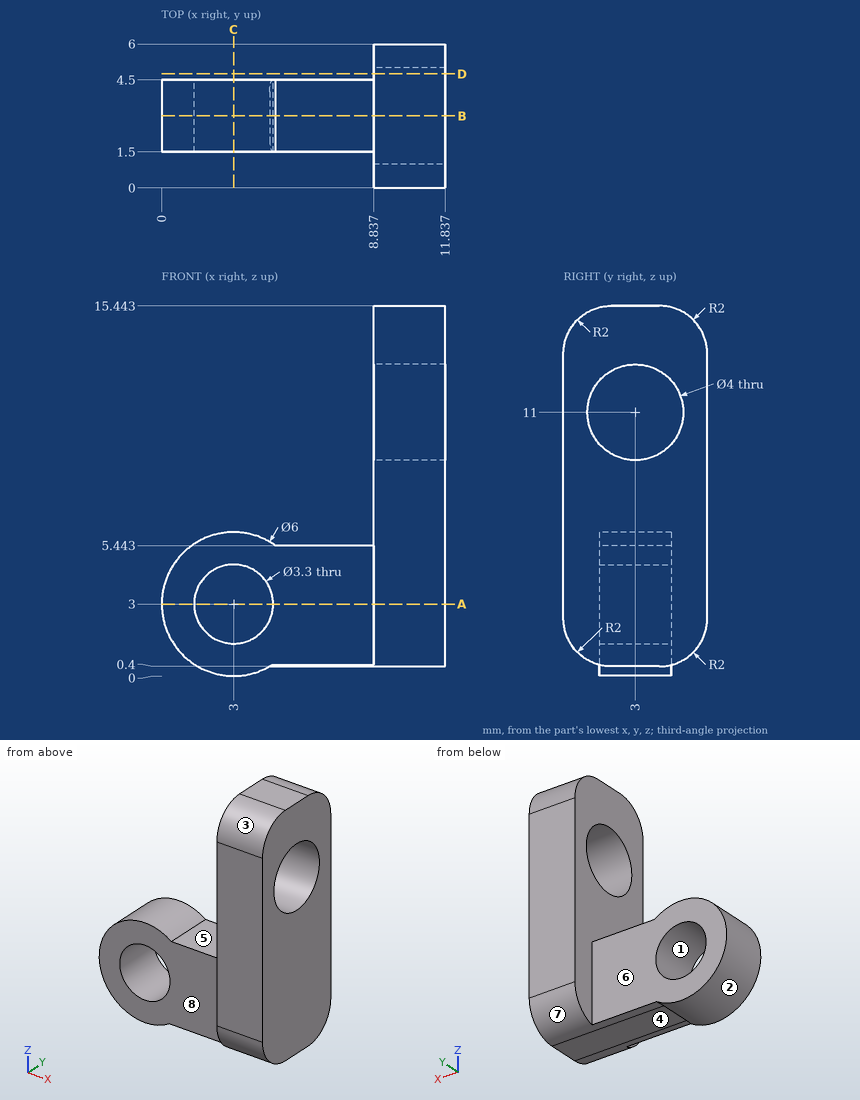
Geometry: see drawing. Coordinates: mm, zero at the bounding-box minimum. A direction names the side the tool comes from. Round coordinates to 2 decimals unless told otherwise and drop trailing zeros. Write each loop counter-clockwise with the first axis right and the second up, starting at its lowest first coordinate (ties: lowest second). Pieces come first, ordered by that corner, then holes. Notation, with made-up numbers: M 39,14 L 63,14 A38 ccw 63,52 Z; hole C 53.5,15 d1. An arc over 180 degrees is marked long. Answer in a Markdown table with one row per item. Add a question column.
(1) Ray query, L1, parallel to Z at x = 3, y = 3; L2, parallel to X at y = 4.25, z = 13; L3, parallel to Z at x = 11.5, y = 2.5. Return the intervals inside material, ascending.
(2) Contact query for flat-ended pins moving along their axis: pin 1 (3 mm diameter, centred on y = 3.5, z = 9, fed in from -X); pin 2 (1 mm diameter, centred on x = 2, y = 3.5, fed in from +Z); pin 3 (1 mm diameter, centred on x = 4, y = 4.5, fed in from -Z). Output: stop coordinate, or through.
(3) Cut plane A-A, the plane z = 3. Return the cut outline in (x, y), then the cut area to 3 significant figures.
(4) Reachability of the marked faces 4, 5, 6, 7 and 8 from +Z, -Z, +X, -X, +Y, -Y: full face, straight path, thin tool, end or side. Return the list, or none.
(5) Cut plane B-B, the plane y = 3. Return the cut outline in (x, z).
(6) Cut plane D-D, the plane y = 4.75. Return the cut outline in (x, z) (1 decimal).
(7) Draft query along Z for the marked faces 1, 2 and 3. Return one class per face: pulls with the +Z half, pulls with the -Z half, needs draft (parallel to the pull), parting line crosses it, or undercut.
(8) Cut plane C-C, the plane x = 3. Return the cut outline in (y, z).
Established:
| question | item | result |
|---|---|---|
| 1 | L1 | 0 to 1.35, 4.65 to 6 |
| 1 | L2 | 8.84 to 11.84 |
| 1 | L3 | 0.4 to 9.06, 12.94 to 15.44 |
| 2 | pin 1 | x = 8.84 |
| 2 | pin 2 | z = 5.96 |
| 2 | pin 3 | z = 0.04 |
| 3 | outline | M 0,1.5 L 1.35,1.5 L 1.35,4.5 L 0,4.5 Z; M 4.65,1.5 L 8.84,1.5 L 8.84,0 L 11.84,0 L 11.84,6 L 8.84,6 L 8.84,4.5 L 4.65,4.5 Z |
| 3 | area | 34.6 mm² |
| 4 | face 4 | -Z, +X, +Y, -Y |
| 4 | face 5 | +Z, +Y, -Y |
| 4 | face 6 | +Z, -Z, -X, +Y |
| 4 | face 7 | -Z, +X, +Y |
| 4 | face 8 | +Z, -Z, -X, -Y |
| 5 | outline | M 4.5,0.4 L 11.84,0.4 L 11.84,9 L 8.84,9 L 8.84,5.44 L 4.74,5.44 A3 ccw long Z; M 8.84,13 L 11.84,13 L 11.84,15.44 L 8.84,15.44 Z; hole C 3,3 d3.3 |
| 6 | outline | M 8.8,0.5 L 11.8,0.5 L 11.8,10 L 8.8,10 Z; M 8.8,12 L 11.8,12 L 11.8,15.3 L 8.8,15.3 Z |
| 7 | face 1 | undercut |
| 7 | face 2 | parting line crosses it |
| 7 | face 3 | pulls with the +Z half |
| 8 | outline | M 1.5,0 L 4.5,0 L 4.5,1.35 L 1.5,1.35 Z; M 1.5,4.65 L 4.5,4.65 L 4.5,6 L 1.5,6 Z |
